Design review of the part built by this model. Coordinates are the model's own, in mm. Give positions to 0.01 mm unless a question says otherwise; leave off trailing zeros. Write each loop counter-clockwise with the first axis right and the second up, starting at its lowest first coordinate (ties: lowest second). Pieces come first, ordered by that corner, then holes. Notation, with made-up numbers: M 9.5,44.5 L 56.5,44.5 A17 ccw 56.5,55.5 Z; hole C 28,-36 d4. An arc over 180 degrees is marked long. Answer in a Markdown table with one row per item.
Autodesk Inventor part; units mm, degrees
ref_plane "YZ Plane" through (0, 0, 0) normal (1, 0, 0) x (0, 1, 0)
ref_plane "XZ Plane" through (0, 0, 0) normal (0, 1, 0) x (-1, 0, 0)
ref_plane "XY Plane" through (0, 0, 0) normal (0, 0, 1) x (1, 0, 0)
sketch "Sketch1" plane through (0, 0, 0) normal (0, 1, 0) x (-1, 0, 0)
  line L0 (-13.5, 3) -> (13.5, 3)
  line L1 (13.5, 3) -> (13.5, -3)
  line L2 (13.5, -3) -> (-13.5, -3)
  line L3 (-13.5, -3) -> (-13.5, 3)
  line L4 (-13.5, 3) -> (13.5, -3) construction
  line L5 (13.5, 3) -> (-13.5, -3) construction
  point P0 (0, 0)
  dimension "d0" = 27
  dimension "d1" = 6
extrude "Extrusion1" add sketch "Sketch1" along normal blind 15
sketch "Sketch2" plane through (0, 15, 0) normal (0, 1, 0) x (1, 0, 0)
  line L0 (-8.5, 0) -> (8.5, 0)
  point P0 (0, 0)
  point P1 (0, 0)
  dimension "d4" = 17
hole "Hole1" at (-8.5, 15, 0) at (8.5, 15, 0) direction (0, -1, 0) diameter 3.3 end through all countersink diameter 6 countersink angle 90
fillet "Fillet1" radius 2 4 edges at (-13.5, 7.5, 3) (-13.5, 7.5, -3) (13.5, 7.5, -3) (13.5, 7.5, 3)
properties part number "FixLock"
1) Add section B-B (y = 7). Write out the cut boundary in (x, z), and give its area (3 significant figures).
Geometry says:
| item | result |
|---|---|
| outline | M -13.5,-1 A2 ccw -11.5,-3 L 11.5,-3 A2 ccw 13.5,-1 L 13.5,1 A2 ccw 11.5,3 L -11.5,3 A2 ccw -13.5,1 Z; hole C -8.5,0 d3.3; hole C 8.5,0 d3.3 |
| area | 141 mm^2 |
2) To check wall thickness, follow probe 1 along X at (y, z) = (5.25, 0); probe 2 along Z at (x, y) = (8.5, 3.5); probe 3 along X at (y, z) = (6, -1.1). State the ranges of each line that lie inside material, in increasing order. Write a range as [from, to].
Geometry says:
| item | result |
|---|---|
| probe 1 | [-13.5, -10.15], [-6.85, 6.85], [10.15, 13.5] |
| probe 2 | [-3, -1.65], [1.65, 3] |
| probe 3 | [-13.5, -9.73], [-7.27, 7.27], [9.73, 13.5] |
3) The part is to be moulded in two halves that separate along Z. For faces 1 (the face through (6.864, 6.729, -0.215)), 2 (the face through (-12.93, 7.6, 2.4)), 3 (the face through (12, 15, 0)), say which applies: released by +Z, released by -Z, zero draft, split by the parting line, or undercut.
Geometry says:
| item | result |
|---|---|
| face 1 | undercut |
| face 2 | released by +Z |
| face 3 | zero draft |
4) Add section A-A (z = 0). Write out the cut boundary in (x, y).
Geometry says:
| item | result |
|---|---|
| outline | M -13.5,0 L -10.15,0 L -10.15,13.65 L -11.5,15 L -13.5,15 Z; M -6.85,0 L 6.85,0 L 6.85,13.65 L 5.5,15 L -5.5,15 L -6.85,13.65 Z; M 10.15,0 L 13.5,0 L 13.5,15 L 11.5,15 L 10.15,13.65 Z |
